```python
from build123d import *

# Parameters (mm, degrees)
SKETCH1_W                              = 350
SKETCH1_H                              = 300
BOSS_EXTRUDE1_DEPTH                    = 20
FILLET1_R                              = 15
SKETCH2_W                              = 100
SKETCH2_H                              = 100
CUT_EXTRUDE1_DEPTH                     = 20
BOSS_EXTRUDE2_DEPTH                    = 10
LPATTERN1_COUNT                        = 2
LPATTERN1_PITCH                        = 110
F_20_0_20_DIAMETER_HOLE2_D             = 20
F_20_0_20_DIAMETER_HOLE2_DEPTH         = 10
F_20_0_20_DIAMETER_HOLE2_CSINK_D       = 20.05
F_20_0_20_DIAMETER_HOLE2_CSINK_ANGLE   = 90
F_20_0_20_DIAMETER_HOLE2_TIP           = 6.00860619
F_18_5_18_5_DIAMETER_HOLE1_D           = 18.5
F_18_5_18_5_DIAMETER_HOLE1_DEPTH       = 10
F_18_5_18_5_DIAMETER_HOLE1_CSINK_D     = 18.55
F_18_5_18_5_DIAMETER_HOLE1_CSINK_ANGLE = 90
F_18_5_18_5_DIAMETER_HOLE1_TIP         = 5.557960726
SKETCH32_W                             = 100
SKETCH32_H                             = 10
BOSS_EXTRUDE3_DEPTH                    = 120
SKETCH37_R                             = 10
CUT_EXTRUDE2_DEPTH                     = 36.07831716
SKETCH45_W                             = 30
SKETCH45_H                             = 65
BOSS_EXTRUDE4_DEPTH                    = 17
M2_5_CLEARANCE_HOLE1_D                 = 2.9
M2_5_CLEARANCE_HOLE1_DEPTH             = 12.4
M2_5_CLEARANCE_HOLE1_CSINK_D           = 2.95
M2_5_CLEARANCE_HOLE1_CSINK_ANGLE       = 90
M2_5_CLEARANCE_HOLE1_TIP               = 0.871247898
SKETCH54_W                             = 10
SKETCH54_H                             = 65
BOSS_EXTRUDE5_DEPTH                    = 17
SKETCH55_W                             = 31
SKETCH55_H                             = 108
BOSS_EXTRUDE6_DEPTH                    = 10
SKETCH59_W                             = 80
SKETCH59_H                             = 20
CUT_EXTRUDE3_DEPTH                     = 21
SKETCH60_W                             = 70
SKETCH60_H                             = 90
CUT_EXTRUDE4_DEPTH                     = 180
SKETCH64_R                             = 3.65
BOSS_EXTRUDE7_DEPTH                    = 10
SKETCH70_R                             = 11
CUT_EXTRUDE5_DEPTH                     = 7
SKETCH75_R                             = 13
SKETCH75_R_2                           = 11
SKETCH75_R_3                           = 3.65
BOSS_EXTRUDE8_DEPTH                    = 8
SKETCH77_R                             = 11
CUT_EXTRUDE6_DEPTH                     = 7


with BuildPart() as part:
    # Sketch1 → Boss-Extrude1 (new body)
    with BuildSketch(Plane(origin=(0, 0, 0), x_dir=(1, 0, 0), z_dir=(0, 1, 0))):
        with Locations((175, -150)):
            Rectangle(SKETCH1_W, SKETCH1_H)
    extrude(amount=BOSS_EXTRUDE1_DEPTH)

    # Fillet1
    fillet1_edges = [part.edges().sort_by_distance(p)[0] for p in [
        (0, 10, 0),
        (350, 10, 0),
        (350, 10, 300),
        (0, 10, 300),
    ]]
    fillet(fillet1_edges, radius=FILLET1_R)

    # Sketch2 → Cut-Extrude1 (cut)
    with BuildSketch(Plane(origin=(0, 20, 0), x_dir=(1, 0, 0), z_dir=(0, 1, 0))):
        with Locations((175, -150)):
            Rectangle(SKETCH2_W, SKETCH2_H)
    extrude(amount=-CUT_EXTRUDE1_DEPTH, mode=Mode.SUBTRACT)

    # Sketch6 → Boss-Extrude2 (add)
    with BuildSketch(Plane.XY.offset(100)):
        with BuildLine():
            Line((125, 0), (125, 130))
            ThreePointArc((125, 130), (175, 180), (225, 130))
            Line((225, 130), (225, 0))
            Line((225, 0), (125, 0))
        make_face()
    boss_extrude2 = extrude(amount=-BOSS_EXTRUDE2_DEPTH)

    # LPattern1: Boss-Extrude2 ×2
    with Locations(*[(0, 0, i * LPATTERN1_PITCH) for i in range(1, LPATTERN1_COUNT)]):
        add(boss_extrude2)

    # Ø20.0 (20) Diameter Hole2
    with Locations(Plane.XY.offset(210)):
        with Locations((175, 155)):
            CounterSinkHole(F_20_0_20_DIAMETER_HOLE2_D / 2, F_20_0_20_DIAMETER_HOLE2_CSINK_D / 2, depth=F_20_0_20_DIAMETER_HOLE2_DEPTH, counter_sink_angle=F_20_0_20_DIAMETER_HOLE2_CSINK_ANGLE)
            with Locations((0, 0, -(F_20_0_20_DIAMETER_HOLE2_DEPTH + F_20_0_20_DIAMETER_HOLE2_TIP / 2))):  # 118° drill point
                Cone(0, F_20_0_20_DIAMETER_HOLE2_D / 2, F_20_0_20_DIAMETER_HOLE2_TIP, mode=Mode.SUBTRACT)

    # Ø18.5 (18.5) Diameter Hole1
    with Locations(Plane(origin=(0, 0, 90), x_dir=(-1, 0, 0), z_dir=(0, 0, -1))):
        with Locations((-175, 155)):
            CounterSinkHole(F_18_5_18_5_DIAMETER_HOLE1_D / 2, F_18_5_18_5_DIAMETER_HOLE1_CSINK_D / 2, depth=F_18_5_18_5_DIAMETER_HOLE1_DEPTH, counter_sink_angle=F_18_5_18_5_DIAMETER_HOLE1_CSINK_ANGLE)
            with Locations((0, 0, -(F_18_5_18_5_DIAMETER_HOLE1_DEPTH + F_18_5_18_5_DIAMETER_HOLE1_TIP / 2))):  # 118° drill point
                Cone(0, F_18_5_18_5_DIAMETER_HOLE1_D / 2, F_18_5_18_5_DIAMETER_HOLE1_TIP, mode=Mode.SUBTRACT)

    # Sketch32 → Boss-Extrude3 (add)
    with BuildSketch(Plane.XY.offset(210)):
        with Locations((175, 125)):
            Rectangle(SKETCH32_W, SKETCH32_H)
    extrude(amount=-BOSS_EXTRUDE3_DEPTH)

    # Sketch37 → Cut-Extrude2 (cut)
    with BuildSketch(Plane(origin=(0, 130, 0), x_dir=(1, 0, 0), z_dir=(0, 1, 0))):
        with Locations((175, -150)):
            Circle(SKETCH37_R)
    extrude(amount=-CUT_EXTRUDE2_DEPTH, mode=Mode.SUBTRACT)

    # Sketch45 → Boss-Extrude4 (add)
    with BuildSketch(Plane(origin=(0, 20, 0), x_dir=(1, 0, 0), z_dir=(0, 1, 0))):
        with Locations((260, -150)):
            Rectangle(SKETCH45_W, SKETCH45_H)
    extrude(amount=BOSS_EXTRUDE4_DEPTH)

    # M2.5 Clearance Hole1
    with Locations(Plane(origin=(0, 37, 0), x_dir=(1, 0, 0), z_dir=(0, 1, 0))):
        with Locations((248.5, -121), (271.5, -121), (271.5, -179), (248.5, -179)):
            CounterSinkHole(M2_5_CLEARANCE_HOLE1_D / 2, M2_5_CLEARANCE_HOLE1_CSINK_D / 2, depth=M2_5_CLEARANCE_HOLE1_DEPTH, counter_sink_angle=M2_5_CLEARANCE_HOLE1_CSINK_ANGLE)
            with Locations((0, 0, -(M2_5_CLEARANCE_HOLE1_DEPTH + M2_5_CLEARANCE_HOLE1_TIP / 2))):  # 118° drill point
                Cone(0, M2_5_CLEARANCE_HOLE1_D / 2, M2_5_CLEARANCE_HOLE1_TIP, mode=Mode.SUBTRACT)

    # Sketch54 → Boss-Extrude5 (add)
    with BuildSketch(Plane(origin=(0, 20, 0), x_dir=(1, 0, 0), z_dir=(0, 1, 0))):
        with Locations((280, -150)):
            Rectangle(SKETCH54_W, SKETCH54_H)
        with Locations((240, -150)):
            Rectangle(SKETCH54_W, SKETCH54_H)
    extrude(amount=BOSS_EXTRUDE5_DEPTH)

    # Sketch55 → Boss-Extrude6 (add)
    with BuildSketch(Plane(origin=(0, 20, 0), x_dir=(1, 0, 0), z_dir=(0, 1, 0))):
        with Locations((317.5, -150)):
            Rectangle(SKETCH55_W, SKETCH55_H)
    extrude(amount=BOSS_EXTRUDE6_DEPTH)

    # Sketch59 → Cut-Extrude3 (cut, through all)
    with BuildSketch(Plane(origin=(0, 20, 0), x_dir=(1, 0, 0), z_dir=(0, 1, 0))):
        with Locations((65, -150)):
            Rectangle(SKETCH59_W, SKETCH59_H)
    extrude(amount=-CUT_EXTRUDE3_DEPTH, mode=Mode.SUBTRACT)

    # Sketch60 → Cut-Extrude4 (cut)
    with BuildSketch(Plane.XY.offset(210)):
        with Locations((175, 65)):
            Rectangle(SKETCH60_W, SKETCH60_H)
    extrude(amount=-CUT_EXTRUDE4_DEPTH, mode=Mode.SUBTRACT)

    # Sketch64 → Boss-Extrude7 (add)
    with BuildSketch(Plane(origin=(0, 0, 0), x_dir=(-1, 0, 0), z_dir=(0, 0, -1))):
        with BuildLine():
            Line((-305, 0), (-305, -15))
            ThreePointArc((-305, -15), (-292, -28), (-279, -15))
            Line((-279, -15), (-279, 0))
            Line((-279, 0), (-305, 0))
        make_face()
        with Locations((-292, -15)):
            Circle(SKETCH64_R, mode=Mode.SUBTRACT)
    extrude(amount=-BOSS_EXTRUDE7_DEPTH)

    # Sketch70 → Cut-Extrude5 (cut)
    with BuildSketch(Plane(origin=(0, 0, 0), x_dir=(-1, 0, 0), z_dir=(0, 0, -1))):
        with Locations((-292, -15)):
            Circle(SKETCH70_R)
    extrude(amount=-CUT_EXTRUDE5_DEPTH, mode=Mode.SUBTRACT)

    # Sketch75 → Boss-Extrude8 (add)
    with BuildSketch(Plane(origin=(0, 0, 0), x_dir=(-1, 0, 0), z_dir=(0, 0, -1))):
        with Locations((-58, -15)):
            Circle(SKETCH75_R)
        with Locations((-58, -15)):
            Circle(SKETCH75_R_2, mode=Mode.SUBTRACT)
        with Locations((-58, -15)):
            Circle(SKETCH75_R_2)
        with Locations((-58, -15)):
            Circle(SKETCH75_R_3, mode=Mode.SUBTRACT)
        with BuildLine():
            Line((-71, 0), (-71, -15))
            ThreePointArc((-71, -15), (-58, -2), (-45, -15))
            Line((-45, -15), (-45, 0))
            Line((-45, 0), (-71, 0))
        make_face()
    extrude(amount=-BOSS_EXTRUDE8_DEPTH)

    # Sketch77 → Cut-Extrude6 (cut)
    with BuildSketch(Plane(origin=(0, 0, 0), x_dir=(-1, 0, 0), z_dir=(0, 0, -1))):
        with Locations((-58, -15)):
            Circle(SKETCH77_R)
    extrude(amount=-CUT_EXTRUDE6_DEPTH, mode=Mode.SUBTRACT)


solid = part.part
```
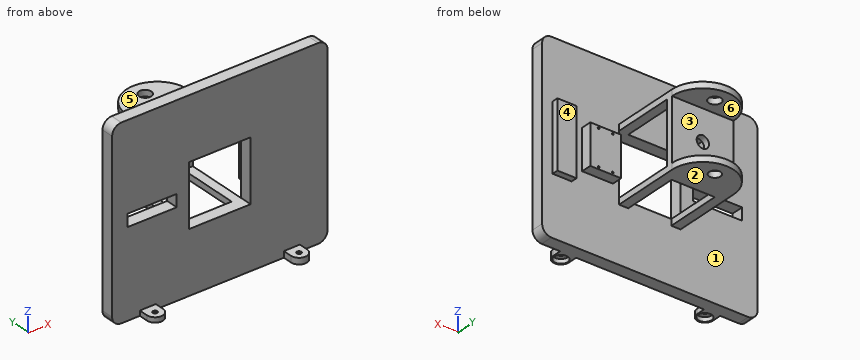
Work out the finished part from the listing and answer in its coordinate system (mm). Face numbers are marked on the shaded views. A direction names the side the tool comes from. Give positions to 0.01 mm unless a question says otherwise; leave off trailing zeros. Loops run counter-clockwise (first coordinate to the right, second up) from the corner with the lowest first, then second, coordinate; pieces in that order, holes last. Notation, with made-up numbers: (61, 83.25) -> (85, 83.25) arc R28 ccw to (85, 107.25) -> close; hole circle Ø3 at (-12, 12.25). An arc over 180 degrees is marked (long way). Write item = value, one per line. Start each with the question number.
(1) The mould has two halves that part along Z. Classify the marked faces 1, 2 and 3: +Z half, -Z half, draft (parallel to the pull), parting line (faces both ways), or undercut.
(2) Find section C-C on y = 6.5. Give the vertices of the cut face in (x, z).
(3) Which of the six approach directions +Z, -Z, +X, -X, +Y, -Y give full straight-line access (tool end or side, diameter ignored) to the marked faces 4, 5 and 6?
(4) Given pin 1 Ø8 at (y, z) = (76, 102.5) entering from +X; pin 2 Ø13.5 at (y, z) = (30.5, 148.5) entering from -X; pin 3 Ø3 at (x, y) = (319, 22.5) entering from -Z, each flat-ended and moving along its own axis, determine where each tip first touches the part or whether it passes through.
(5) Find section A-A on z = 134. Give the vertices of the cut face in (x, y), and give its area (3 significant figures).
(6) Find section D-D on x = 327.5. Give the vertices of the cut face in (y, z).
(7) Find the intervals of material crossed by probe 1 along X at (y, z) = (29.5, 179); probe 2 along Z at (x, y) = (271.5, 29); probe 3 along X at (y, z) = (33.75, 179), in increasing order. Write a range as from..to.
(8) Find section B-B on y = 79. Give the vertices of the cut face in (x, z).
From the geometry:
q1.face_1 = draft
q1.face_2 = -Z half
q1.face_3 = undercut
q2.outline = (0, 15) arc R15 ccw to (15, 0) -> (335, 0) arc R15 ccw to (350, 15) -> (350, 285) arc R15 ccw to (335, 300) -> (15, 300) arc R15 ccw to (0, 285) -> close; hole (25, 140) -> (105, 140) -> (105, 160) -> (25, 160) -> close; hole (125, 100) -> (225, 100) -> (225, 200) -> (125, 200) -> close
q3.face_4 = +Z, -Z, +X, +Y
q3.face_5 = +Z, +X, -X, +Y
q3.face_6 = +X, -X, +Y
q4.pin_1 = 225
q4.pin_2 = 235
q4.pin_3 = 96
q5.outline = (0, 0) -> (125, 0) -> (125, 20) -> (0, 20) -> close; (125, 120) -> (225, 120) -> (225, 130) -> (125, 130) -> close; (225, 0) -> (350, 0) -> (350, 20) -> (333, 20) -> (333, 30) -> (302, 30) -> (302, 20) -> (285, 20) -> (285, 37) -> (235, 37) -> (235, 20) -> (225, 20) -> close
q5.area = 7,160 mm^2
q6.outline = (0, 0) -> (20, 0) -> (20, 96) -> (30, 96) -> (30, 204) -> (20, 204) -> (20, 300) -> (0, 300) -> close
q7.probe_1 = 235..247.05, 249.95..270.05, 272.95..285, 302..333
q7.probe_2 = 117.5..119.55, 122.45..177.55, 180.45..182.5
q7.probe_3 = 235..247.05, 249.95..270.05, 272.95..285
q8.outline = (125, 90) -> (140, 90) -> (140, 100) -> (125, 100) -> close; (125, 200) -> (140, 200) -> (140, 210) -> (125, 210) -> close; (210, 90) -> (225, 90) -> (225, 100) -> (210, 100) -> close; (210, 200) -> (225, 200) -> (225, 210) -> (210, 210) -> close
